Geometry: see drawing. Coordinates: mm, zero at the bounding-box minimum. Round coordinates to 2 decimals unless told otherwise and drop trailing zeros. Write each loop counter-clockwise with the first axis right and the second up, starting at its lowest first coordinate (ties: lowest second). Pieces come first, ordered by that corner, then holes. Notation, with made-up numbers: (-1.5, 53.25) -> (51.5, 53.25) arc R25 ccw to (51.5, 90.25) -> close; hole circle Ø5 at (39.25, 62). An arc over 180 degrees is marked (long way). Write item = value, one per line. Start each with the question number.
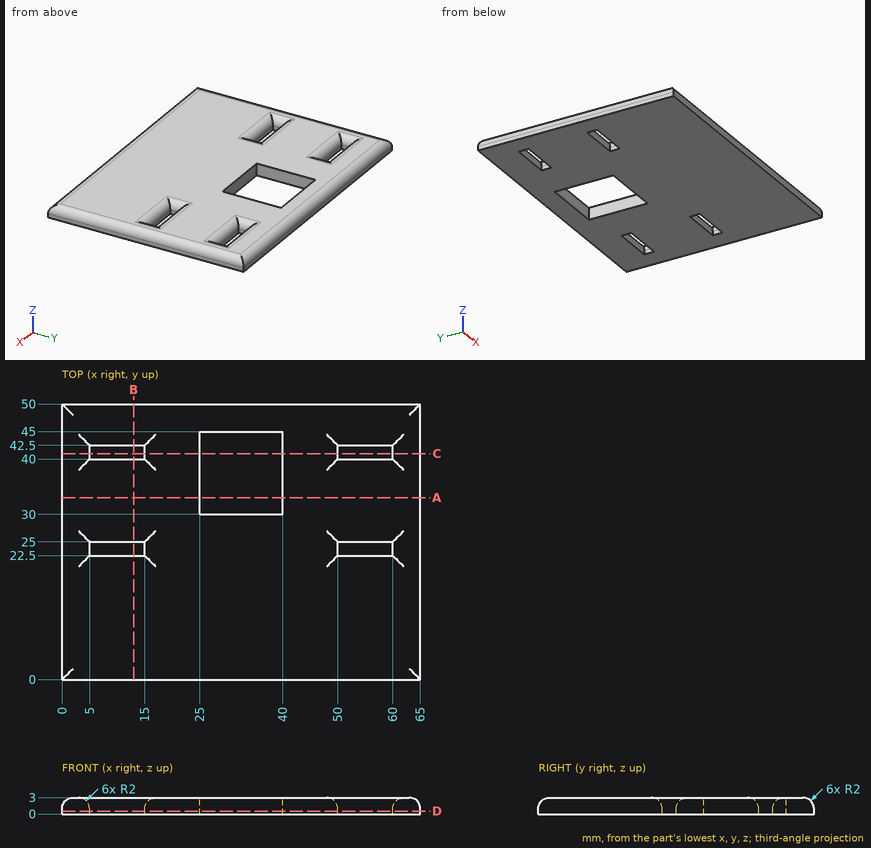
1. Section A-A (y = 33). Output: boundary loops of the cut face in (x, z).
2. Pin query (flat end, axial travel): P1, Ø1, axis at x = 47, z = 2, coming from the +Y side; P2, Ø1.5, axis at y = 32.5, z = 2.5, coming from the -X side. Return the tip coordinate at first contact, or that it passes through.
3. Section D-D (z = 0.55). Output: boundary loops of the cut face in (x, y).
4. Section C-C (y = 41). Output: boundary loops of the cut face in (x, z), then the cut area to 3 significant figures.
5. Line query: line 1 along Y through (x, z) = (10.5, 0.2); line 2 along Y through (x, z) = (56, 2.7); line 3 along Y through (x, z) = (39.5, 0.95). Output: solid intervals per line, ascending.
6. Section B-B (x = 13). Output: boundary loops of the cut face in (y, z).
Check sheet entries:
q1.outline = (0, 0) -> (25, 0) -> (25, 3) -> (2, 3) arc R2 ccw to (0, 1) -> close; (40, 0) -> (65, 0) -> (65, 1) arc R2 ccw to (63, 3) -> (40, 3) -> close
q2.P1 = 49.94
q2.P2 = 0.15
q3.outline = (0, 0) -> (65, 0) -> (65, 50) -> (0, 50) -> close; hole (5, 22.5) -> (15, 22.5) -> (15, 25) -> (5, 25) -> close; hole (5, 40) -> (15, 40) -> (15, 42.5) -> (5, 42.5) -> close; hole (25, 30) -> (40, 30) -> (40, 45) -> (25, 45) -> close; hole (50, 22.5) -> (60, 22.5) -> (60, 25) -> (50, 25) -> close; hole (50, 40) -> (60, 40) -> (60, 42.5) -> (50, 42.5) -> close
q4.outline = (0, 0) -> (5, 0) -> (5, 1) arc R2 ccw to (3, 3) -> (2, 3) arc R2 ccw to (0, 1) -> close; (15, 0) -> (25, 0) -> (25, 3) -> (17, 3) arc R2 ccw to (15, 1) -> close; (40, 0) -> (50, 0) -> (50, 1) arc R2 ccw to (48, 3) -> (40, 3) -> close; (60, 0) -> (65, 0) -> (65, 1) arc R2 ccw to (63, 3) -> (62, 3) arc R2 ccw to (60, 1) -> close
q4.area = 84.8 mm2
q5.line_1 = 0 to 22.5, 25 to 40, 42.5 to 50
q5.line_2 = 0.95 to 21.55, 25.95 to 39.05, 43.45 to 49.05
q5.line_3 = 0 to 30, 45 to 50
q6.outline = (0, 0) -> (22.5, 0) -> (22.5, 1) arc R2 ccw to (20.5, 3) -> (2, 3) arc R2 ccw to (0, 1) -> close; (25, 0) -> (40, 0) -> (40, 1) arc R2 ccw to (38, 3) -> (27, 3) arc R2 ccw to (25, 1) -> close; (42.5, 0) -> (50, 0) -> (50, 1) arc R2 ccw to (48, 3) -> (44.5, 3) arc R2 ccw to (42.5, 1) -> close
